from build123d import *

# Parameters (mm, degrees)
SKETCH1_W           = 35.56
SKETCH1_H           = 35.56
BOSS_EXTRUDE1_DEPTH = 73.5965
SKETCH2_R           = 4.7625
CUT_EXTRUDE1_DEPTH  = 84.648591215
SKETCH3_W           = 25.4
SKETCH3_H           = 35.56
BOSS_EXTRUDE2_DEPTH = 44.45
SKETCH5_W           = 25.4
SKETCH5_H           = 44.45
BOSS_EXTRUDE3_DEPTH = 6.35
SKETCH6_W           = 25.4
SKETCH6_H           = 44.45
BOSS_EXTRUDE4_DEPTH = 6.35
SKETCH4_R           = 17.500000052
CUT_EXTRUDE2_DEPTH  = 84.232998938
SKETCH8_W           = 11.185009969
SKETCH8_H           = 15.24
CUT_EXTRUDE3_DEPTH  = 7.62
SKETCH9_W           = 48.26
SKETCH9_H           = 44.45
BOSS_EXTRUDE6_DEPTH = 3.81
SKETCH12_W          = 8.37609249
SKETCH12_H          = 15.24
CUT_EXTRUDE5_DEPTH  = 3.81
SKETCH13_R          = 5.588
CUT_EXTRUDE6_DEPTH  = 3.81
SKETCH14_R          = 1.5
CUT_EXTRUDE7_DEPTH  = 3.81


with BuildPart() as part:
    # Sketch1 → Boss-Extrude1 (new body)
    with BuildSketch(Plane(origin=(0, 0, 0), x_dir=(1, 0, 0), z_dir=(0, 1, 0))):
        Rectangle(SKETCH1_W, SKETCH1_H)
    extrude(amount=-BOSS_EXTRUDE1_DEPTH)

    # Sketch2 → Cut-Extrude1 (cut, through all)
    with BuildSketch(Plane.XY.offset(17.78)):
        with Locations((0, -19.05)):
            Circle(SKETCH2_R)
        with Locations((0, -36.83)):
            Circle(SKETCH2_R)
        with Locations((0, -55.88)):
            Circle(SKETCH2_R)
    extrude(amount=-CUT_EXTRUDE1_DEPTH, mode=Mode.SUBTRACT)

    # Sketch3 → Boss-Extrude2 (add)
    with BuildSketch(Plane(origin=(0, 0, 0), x_dir=(1, 0, 0), z_dir=(0, 1, 0))):
        Rectangle(SKETCH3_W, SKETCH3_H)
    extrude(amount=BOSS_EXTRUDE2_DEPTH)

    # Sketch5 → Boss-Extrude3 (add)
    with BuildSketch(Plane.XY.offset(17.78)):
        with Locations((0, 22.225)):
            Rectangle(SKETCH5_W, SKETCH5_H)
    extrude(amount=BOSS_EXTRUDE3_DEPTH)

    # Sketch6 → Boss-Extrude4 (add)
    with BuildSketch(Plane(origin=(0, 0, -17.78), x_dir=(-1, 0, 0), z_dir=(0, 0, -1))):
        with Locations((0, 22.225)):
            Rectangle(SKETCH6_W, SKETCH6_H)
    extrude(amount=BOSS_EXTRUDE4_DEPTH)

    # Sketch4 → Cut-Extrude2 (cut, through all)
    with BuildSketch(Plane(origin=(12.7, 0, 0), x_dir=(0, 0, -1), z_dir=(1, 0, 0))):
        with Locations((0, 22.225)):
            Circle(SKETCH4_R)
    extrude(amount=-CUT_EXTRUDE2_DEPTH, mode=Mode.SUBTRACT)

    # Sketch8 → Cut-Extrude3 (cut)
    with BuildSketch(Plane.ZY.offset(12.7)):
        with Locations((-18.537495016, 22.225)):
            Rectangle(SKETCH8_W, SKETCH8_H)
    extrude(amount=-CUT_EXTRUDE3_DEPTH, mode=Mode.SUBTRACT)

    # Sketch9 → Boss-Extrude6 (add)
    with BuildSketch(Plane.ZY.offset(12.7)):
        with Locations((0, 22.225)):
            Rectangle(SKETCH9_W, SKETCH9_H)
    extrude(amount=BOSS_EXTRUDE6_DEPTH)

    # Sketch12 → Cut-Extrude5 (cut)
    with BuildSketch(Plane(origin=(-12.7, 0, 0), x_dir=(0, 0, -1), z_dir=(1, 0, 0))):
        with Locations((19.941953755, 22.225)):
            Rectangle(SKETCH12_W, SKETCH12_H)
    extrude(amount=-CUT_EXTRUDE5_DEPTH, mode=Mode.SUBTRACT)

    # Sketch13 → Cut-Extrude6 (cut)
    with BuildSketch(Plane.ZY.offset(16.51)):
        with Locations((0, 21.902286104)):
            Circle(SKETCH13_R)
    extrude(amount=-CUT_EXTRUDE6_DEPTH, mode=Mode.SUBTRACT)

    # Sketch14 → Cut-Extrude7 (cut)
    with BuildSketch(Plane.ZY.offset(16.51)):
        with Locations((-6.604, 28.956)):
            Circle(SKETCH14_R)
        with Locations((-8.89, 13.462)):
            Circle(SKETCH14_R)
        with Locations((8.89, 30.988)):
            Circle(SKETCH14_R)
        with Locations((6.604, 15.494)):
            Circle(SKETCH14_R)
    extrude(amount=-CUT_EXTRUDE7_DEPTH, mode=Mode.SUBTRACT)


solid = part.part
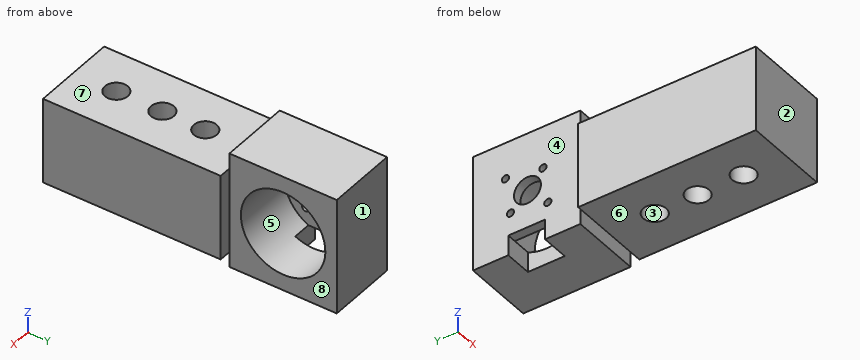
The model under review builds one solid part; all positions refer to its coordinate system, in mm. Face numbers are marked on the shaded views. A direction names the side the tool comes from. Give positions to 0.01 mm unless a question says otherwise; leave off trailing zeros. Order: outer loops, then holes, each group sorted by start corner. A loop starts at its lowest first (then second) coordinate and runs counter-clockwise, first axis right, second up. Notation, with made-up numbers: (68.25, 43.5) -> (115.25, 43.5) arc R7 cw to (115.25, 49.5) -> close; hole circle Ø5 at (-12, -34.75). An arc over 180 degrees is marked (long way). Write item = value, one per line. Start each with the question number.
(1) Tool access review of the marked faces 5, 6, 7 and 8: name each direction out of +Z, -Z, +X, -X, +Y, -Y from which nothing blocks a thin tool from reaching the whole face with its end or side.
(2) Take a section at A-A (y = -36.83). Write out the cut boundary in (x, z), plus the area to 3 significant figures.
(3) For L1, parallel to Y at x = -14.5, z = -0.5; L2, parallel to X at y = -36.5, z = -12; L3, parallel to Y at x = 3, z = 1, list the stretches that pass through material, from the lowest coordinate up. Write a range as from..to.
(4) Take a section at B-B (x = 3.5). State how many separate pieces and enclosed holes the cut face has, plus the area to 3 significant figures.
(5) For pin 1 Ø5 at (y, z) = (15.494, 6.604) entering from -X; pin 2 Ø15 at (x, y) = (0, -55.88) entering from +Z; pin 3 Ø1 at (y, z) = (12.5, -12) entering from +X, all flat-tipped, find the tip position at first contact; note any pin that passes through.
(6) Draft analysis for pull direction Y (two halves, no side actions). For the marked faces 1, 2, 3 and 4, state which applies: +Y half, -Y half, draft (parallel to the pull), parting line (faces both ways), or undercut.
Returned:
q1.face_5 = +X
q1.face_6 = -Z, +X, -X, -Y
q1.face_7 = +Z, +X, -X, -Y
q1.face_8 = +Z, -Z, +X, +Y
q2.outline = (-17.78, -17.78) -> (-4.76, -17.78) -> (-4.76, 17.78) -> (-17.78, 17.78) -> close; (4.76, -17.78) -> (17.78, -17.78) -> (17.78, 17.78) -> (4.76, 17.78) -> close
q2.area = 926 mm²
q3.L1 = -73.6..16.34, 27.47..44.45
q3.L2 = -17.78..-4.75, 4.75..17.78
q3.L3 = -73.6..-59.58, -52.18..-40.53, -33.13..-22.75, -15.35..4.75, 39.7..44.45
q4.separate_pieces = 4
q4.enclosed_holes = 1
q4.area = 3,110 mm²
q5.pin_1 = -16.51
q5.pin_2 = 17.78
q5.pin_3 = -12.7
q6.face_1 = +Y half
q6.face_2 = -Y half
q6.face_3 = undercut
q6.face_4 = draft
